The listing builds one solid part. Answer for the finished solid, in the listing's coordinates (mm). Face numbers are marked on the shaded views. Round coordinates to 2 decimals unless told otherwise and drop trailing zeros. Order: outer loops, then holes, each group sorted by start corner. A loop starts at its lowest first (then second) coordinate and runs counter-clockwise, first axis right, second up. Notation, with made-up numbers: (17, -2) -> (22, -2) arc R14 cw to (22, 14) -> close; hole circle Ø7 at (-1, 2.25). An arc over 180 degrees is marked (long way). Return JSON: item names as keys, results as strings. Group by question number.
(1) Each of these flat-tipped pins is pushed along its axis until it touches: pin 1 (5 mm diameter, centred on x = -9, z = 5, fed in from -Y); pin 2 (3 mm diameter, centred on x = -7.5, z = 4.5, fed in from +Y). Where does it stop, or does it pass through?
(2) Determine the mould class of the marked faces 1, 2 and 3 for opening direction Y: +Y half, -Y half, draft (parallel to the pull), parting line (faces both ways), or undercut.
(3) The part is cut by section C-C (z = 3.75). Determine the outline of the cut face in (x, y).
(4) Consider line 1 (Y direction, x = 0, z = 4.5); line 2 (Y direction, x = -13.5, z = 7.75); line 3 (X direction, y = -15, z = 6.75). Determine where each line is inside the solid, lowest interval first. Write a range as [from, to].
(5) The part is cut by section B-B (y = 17.5). Determine the outline of the cut face in (x, z).
(6) The part is cut by section A-A (x = 0). Determine the outline of the cut face in (y, z), plus the area to 3 significant figures.
from build123d import *

# Parameters (mm, degrees)
SKETCH_R        = 27.5
SKETCH_R_2      = 19.5
PAD_DEPTH       = 10
SKETCH001_R     = 1.5
POCKET_DEPTH    = 10
SKETCH002_R     = 1.5
POCKET001_DEPTH = 1.5


with BuildPart() as part:
    # Sketch → Pad (new body)
    with BuildSketch(Plane.XY):
        Circle(SKETCH_R)
        Circle(SKETCH_R_2, mode=Mode.SUBTRACT)
    extrude(amount=PAD_DEPTH)

    # Sketch001 → Pocket (cut)
    with BuildSketch(Plane(origin=(27.5, 0, 0), x_dir=(1, 0, 0), z_dir=(0, 0, 1))):
        Circle(SKETCH001_R)
    extrude(amount=POCKET_DEPTH, mode=Mode.SUBTRACT)

    # Sketch002 → Pocket001 (cut)
    with BuildSketch(Plane.YZ.offset(27.5)):
        Circle(SKETCH002_R)
    extrude(amount=-POCKET001_DEPTH, mode=Mode.SUBTRACT)


solid = part.part
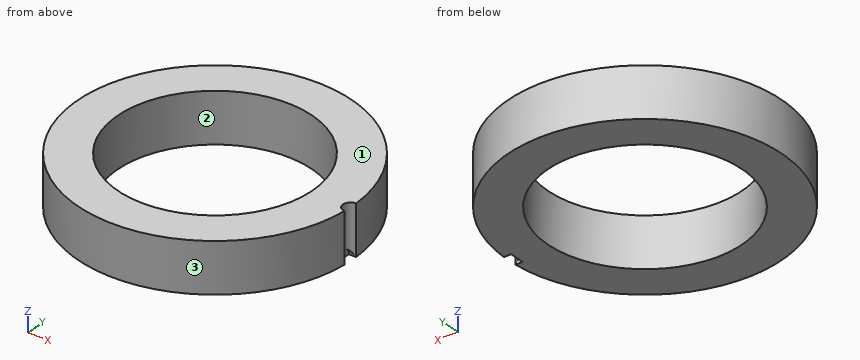
Answer below:
{
 "1": {"pin 1": "stops at y = -26.72", "pin 2": "stops at y = 26.84"},
 "2": {"face 1": "draft", "face 2": "undercut", "face 3": "parting line"},
 "3": {"outline": "(27.46, -1.5) arc R1.5 cw to (27.46, 1.5) arc R27.5 ccw (long way) to start; hole circle Ø39 at (0, 0)"},
 "4": {"line 1": "y = [-27.5, -19.5], [19.5, 27.5]", "line 2": "y = [-23.96, -14.07], [14.07, 23.96]", "line 3": "x = [-23.05, -12.46], [12.46, 23.05]"},
 "5": {"outline": "(-21.21, 0) -> (-8.6, 0) -> (-8.6, 10) -> (-21.21, 10) -> close; (8.6, 0) -> (21.21, 0) -> (21.21, 10) -> (8.6, 10) -> close"},
 "6": {"outline": "(-27.5, 0) -> (-19.5, 0) -> (-19.5, 10) -> (-27.5, 10) -> close; (19.5, 0) -> (27.5, 0) -> (27.5, 10) -> (19.5, 10) -> close", "area": "160 mm²"}
}
